Can you work these out from the model? Positions are in its coordinate system, mm. A direction names the side the tool comes from. Give positions to 0.01 mm unless a question says otherwise; leave off trailing zeros. Write each loop counter-clockwise with the first axis right and the second up, starting at its lowest first coordinate (ties: lowest second). Pieces come first, ordered by that corner, then holes.
from build123d import *

# Parameters (mm, degrees)
F0_W     = 123.8177604973
F0_H     = 36.5064647049
F1_DEPTH = 5.08
F2_DEPTH = 4.826
F3_W     = 123.8177604973
F3_H     = 3.7974044681
F4_DEPTH = 6.35
F5_W     = 123.8177604973
F5_H     = 5.0793443806
F6_DEPTH = 36.068
F7_SIZE  = 5.079


# Not quite as in the source:
# - a fillet or chamfer is up to 0.001 mm smaller than in the source, because OpenCascade refuses the exact size


with BuildPart() as f1:
    # F0 (on Front) → F1 (new body)
    with BuildSketch(Plane.XZ):
        with Locations((4.7154184431, 8.8223954663)):
            Rectangle(F0_W, F0_H)
    extrude(amount=F1_DEPTH)

    # F0 (on Front) → F2 (join)
    with BuildSketch(Plane.XZ):
        with Locations((4.7154184431, 8.8223954663)):
            Rectangle(F0_W, F0_H)
    extrude(amount=F2_DEPTH)

    # F3 (on face) → F4 (join)
    with BuildSketch(Plane.XZ.offset(5.08)):
        with Locations((4.7154184431, 25.1769255847)):
            Rectangle(F3_W, F3_H)
    extrude(amount=F4_DEPTH)

    # F5 (on face) → F6 (join)
    with BuildSketch(Plane.XZ.offset(5.08)):
        with Locations((4.7154184431, -6.8911646958)):
            Rectangle(F5_W, F5_H)
    extrude(amount=F6_DEPTH)

    # F7 (size 5.08 in the source; OpenCascade refuses exactly that, so slightly less here)
    f7_edges = [f1.edges().sort_by_distance(p)[0] for p in [
        (4.715418, -41.148, -4.351493),
    ]]
    chamfer(f7_edges, length=F7_SIZE)


solid = f1.part
(1) For faces 1 (the face through (4, -8, 23.278)), 2 (the face through (4, -11.43, 25)), 3 (the face through (4, -6, 27.076)), which set-ups out of +Z, -Z, +X, -X, +Y, -Y let a thin tool reach every point of the face, with its end or its side?
Returned:
face 1: +X, -X, -Y
face 2: +Z, +X, -X, -Y
face 3: +Z, +X, -X, +Y, -Y
(2) Will these pins go through, and if not, where does the flat tip stop? P1, Ø4, axis at x = 41.5, z = 14.5, coming from the -Y side; P2, Ø4, axis at x = 45.5, z = 16.5, coming from the +Y side; P3, Ø12, axis at x = 47.5, y = -31, coming from the +Z side; P4, Ø1.9, axis at x = 34.5, z = 25.5, coming from the -Y side.
Returned:
P1: stops at y = -5.08
P2: stops at y = 0
P3: stops at z = -4.35
P4: stops at y = -11.43
(3) Imagine slicing it at D-D, the plane y = -29. Write out the boundary of the cut face in (x, z), plus the area to 3 significant figures.
Returned:
outline: (-57.19, -9.43) - (66.62, -9.43) - (66.62, -4.35) - (-57.19, -4.35) - close
area: 629 mm2
(4) If we mould it in two halves opening along Z, with no side actions, what happens to faces 4 (the face through (4, -20, -9.431)), 5 (the face through (4, -5.08, 10)), 6 (the face through (-57.193, -13, -5)), 7 (the face through (3.849, -38.644, -6.927))? For each: +Z half, -Z half, draft (parallel to the pull), parting line (faces both ways), or undercut.
Returned:
face 4: -Z half
face 5: undercut
face 6: draft
face 7: +Z half
(5) Imagine slicing it at C-C, the plane z = 7. Write out the boundary of the cut face in (x, y), plus the area to 3 significant figures.
Returned:
outline: (-57.19, -5.08) - (66.62, -5.08) - (66.62, 0) - (-57.19, 0) - close
area: 629 mm2
(6) If I drill on L1, parallel to Z at x = 48, y = -6; L2, parallel to Z at x = -52, y = -26; L3, parallel to Y at x = -24, z = -2, over which ranges is the centre line in solid material (lowest first)?
Returned:
L1: z = -9.43 to -4.35, 23.28 to 27.08
L2: z = -9.43 to -4.35
L3: y = -5.08 to 0
(7) Imagine slicing it at A-A, the plane y = -9. Write out the boundary of the cut face in (x, z), plus the area to 3 significant figures.
Returned:
outline: (-57.19, -9.43) - (66.62, -9.43) - (66.62, -4.35) - (-57.19, -4.35) - close; (-57.19, 23.28) - (66.62, 23.28) - (66.62, 27.08) - (-57.19, 27.08) - close
area: 1,100 mm2
